from build123d import *

# Parameters (mm, degrees)
SKETCH1_W           = 501.65
SKETCH1_H           = 349.25
BOSS_EXTRUDE1_DEPTH = 9.525
SKETCH2_R           = 3.175
CUT_EXTRUDE1_DEPTH  = 9.525
SKETCH4_R           = 3.571875
CUT_EXTRUDE2_DEPTH  = 9.525
CHAMFER1_SIZE       = 2.921
CHAMFER1_SIZE2      = 2.630080213
CUT_EXTRUDE3_DEPTH  = 9.525


with BuildPart() as part:
    # Sketch1 → Boss-Extrude1 (new body)
    with BuildSketch(Plane(origin=(0, 0, 0), x_dir=(1, 0, 0), z_dir=(0, 1, 0))):
        with Locations((259.3132527, -174.625)):
            Rectangle(SKETCH1_W, SKETCH1_H)
    extrude(amount=BOSS_EXTRUDE1_DEPTH)

    # Sketch2 → Cut-Extrude1 (cut)
    with BuildSketch(Plane(origin=(0, 9.525, 0), x_dir=(1, 0, 0), z_dir=(0, 1, 0))):
        with Locations((392.6632527, -338.1375)):
            Circle(SKETCH2_R)
        with Locations((151.3632527, -338.1375)):
            Circle(SKETCH2_R)
        with Locations((367.2632527, -11.1125)):
            Circle(SKETCH2_R)
        with Locations((125.9632527, -11.1125)):
            Circle(SKETCH2_R)
        with Locations((19.6007527, -250.825)):
            Circle(SKETCH2_R)
        with Locations((19.6007527, -98.425)):
            Circle(SKETCH2_R)
        with Locations((499.0257527, -250.825)):
            Circle(SKETCH2_R)
        with Locations((499.0257527, -98.425)):
            Circle(SKETCH2_R)
    extrude(amount=-CUT_EXTRUDE1_DEPTH, mode=Mode.SUBTRACT)

    # Sketch4 → Cut-Extrude2 (cut)
    with BuildSketch(Plane(origin=(0, 9.525, 0), x_dir=(1, 0, 0), z_dir=(0, 1, 0))):
        with Locations((472.0382527, -38.1)):
            Circle(SKETCH4_R)
        with Locations((472.0382527, -311.15)):
            Circle(SKETCH4_R)
        with Locations((46.5882527, -311.15)):
            Circle(SKETCH4_R)
        with Locations((46.5882527, -38.1)):
            Circle(SKETCH4_R)
    extrude(amount=-CUT_EXTRUDE2_DEPTH, mode=Mode.SUBTRACT)

    # Chamfer1
    chamfer1_edges = [part.edges().sort_by_distance(p)[0] for p in [
        (43.0163777, 0, 38.1),
        (43.0163777, 0, 311.15),
        (468.4663777, 0, 311.15),
        (468.4663777, 0, 38.1),
    ]]
    chamfer1_side = [part.faces().sort_by_distance(p)[0] for p in [
        (259.3132527, 0, 174.625),
    ]]
    chamfer(chamfer1_edges, length=CHAMFER1_SIZE, length2=CHAMFER1_SIZE2, reference=chamfer1_side[0])

    # Sketch5 → Cut-Extrude3 (cut)
    with BuildSketch(Plane(origin=(0, 9.525, 0), x_dir=(1, 0, 0), z_dir=(0, 1, 0))):
        Polygon((37.3137367, 0), (8.4882527, -28.825484), (8.4882527, 0), align=None)
        Polygon((510.1382527, -28.825484), (510.1382527, 0), (481.3127687, 0), align=None)
        Polygon((481.3127687, -349.25), (510.1382527, -320.424516), (510.1382527, -349.25), align=None)
        Polygon((8.4882527, -320.424516), (8.4882527, -349.25), (37.3137367, -349.25), align=None)
    extrude(amount=-CUT_EXTRUDE3_DEPTH, mode=Mode.SUBTRACT)


solid = part.part
Verification items for the finished model (mm, model axes). Give positions to 0.01 mm unless a question says otherwise; leave off trailing zeros. Write item = value, one per line. Start each with the question number.
Q1. Thickness scan on line 1 (X direction, y = 5.75, z = 38.1); line 2 (Z direction, x = 46, y = 1.25); line 3 (X direction, y = 8, z = 322.5). Record the ranges inside material, lowest first.
Q2. Mould release check, pull along Z, two halves, no side actions. Record for faces 1 (the face through (468.328, 2.502, 37.937)), 2 (the face through (495.52, 4.83, 14.21)), 3 (the face through (256, 9.525, 172)): released by +Z, released by -Z, zero draft, split by the parting line, or undercut.
Q3. Depth check by flat-ended pin: P1, Ø9.5, axis at x = 46.59, z = 38.1, coming from the -Y side. Enter the tip coordinate at first touch or a pass-through.
Answer key:
q1.line_1 = 8.49 to 43.02, 50.16 to 468.47, 475.61 to 510.14
q1.line_2 = 0 to 33.03, 43.17 to 306.08, 316.22 to 349.25
q1.line_3 = 10.56 to 508.06
q2.face_1 = undercut
q2.face_2 = released by -Z
q2.face_3 = zero draft
q3.P1 = 1.57
